Read the model definition and answer for the solid it produces. Units are mm, in the model's axes. Face numbers are marked on the shaded views. A direction names the side the tool comes from. Give positions to 0.01 mm unless a question says otherwise; leave off trailing zeros. Loops run counter-clockwise (first coordinate to the right, second up) from the corner with the lowest first, then second, coordinate; pieces in that order, holes last.
(1) Which of the six approach directions +Z, -Z, +X, -X, +Y, -Y give full straight-line access (tool end or side, diameter ignored) to the marked faces 1 and 2?
(2) Find section A-A, the plane z = 0. Write down the section's boundary in (x, y), then the cut area to 3 significant figures.
(3) Find section D-D, the plane x = 20. Write down the section's boundary in (y, z), then the cut area to 3 significant figures.
(4) Find section B-B, the plane x = 0. Write down the section's boundary in (y, z), then the cut area to 3 significant figures.
(5) Straight lines are drawn through the part: probe 1 along Y at (x, z) = (-24, -19); probe 2 along X at (y, z) = (8, 3.5); probe 3 along X at (y, z) = (8, -10). For each, find the intervals that lie inside material, in ascending order.
(6) Find section C-C, the plane y = 7.5. Write down the section's boundary in (x, z), then the cut area to 3 significant figures.
(7) This flat-tipped pin is pushed along its axis until it touches: P1, Ø2, axis at x = -23.5, z = -9.5, coming from the +Y side. Where does it stop, or does it pass through?
```python
from build123d import *

# Parameters (mm, degrees)
F0_W     = 65.434128046
F0_H     = 41.7352281511
F1_DEPTH = 25.4
F2_R     = 15.9425701821
F3_DEPTH = 7.366
F4_DEPTH = 0.254
F5_DEPTH = 3.302


with BuildPart() as f1:
    # F0 (on Front) → F1 (new body)
    with BuildSketch(Plane.XZ):
        Rectangle(F0_W, F0_H)
    extrude(amount=F1_DEPTH)

    # F2 (on face) → F3 (join)
    with BuildSketch(Plane(origin=(0, 0, 0), x_dir=(-1, 0, 0), z_dir=(0, 1, 0))):
        Circle(F2_R)
    extrude(amount=F3_DEPTH)

    # F4 (add): a face of the model
    f4_faces = [f1.faces().sort_by_distance(p)[0] for p in [
        (31.9409548566, 0, 0),
    ]]
    extrude(f4_faces, amount=F4_DEPTH)

    # F5 (add): a face of the model
    f5_faces = [f1.faces().sort_by_distance(p)[0] for p in [
        (0, 7.366, 0),
    ]]
    extrude(f5_faces, amount=F5_DEPTH)


solid = f1.part
```
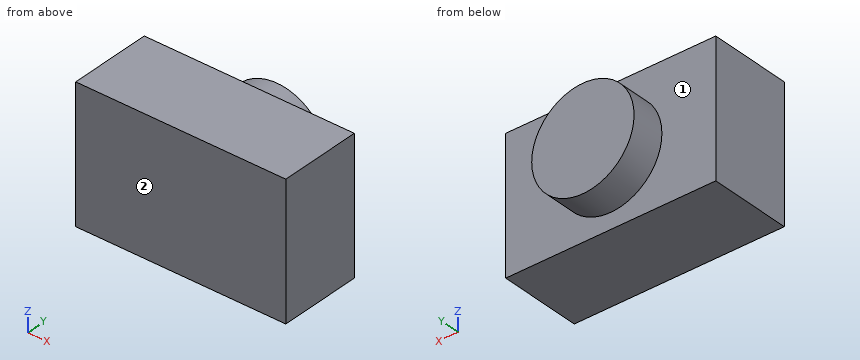
Entries:
1. face 1: +Y
1. face 2: +Z, -Z, +X, -X, -Y
2. outline: (-32.72, -25.4) - (32.72, -25.4) - (32.72, 0.25) - (15.94, 0.25) - (15.94, 10.67) - (-15.94, 10.67) - (-15.94, 0.25) - (-32.72, 0.25) - close
2. area: 2,010 mm2
3. outline: (-25.4, -20.87) - (0.25, -20.87) - (0.25, 20.87) - (-25.4, 20.87) - close
3. area: 1,070 mm2
4. outline: (-25.4, -20.87) - (0.25, -20.87) - (0.25, -15.94) - (10.67, -15.94) - (10.67, 15.94) - (0.25, 15.94) - (0.25, 20.87) - (-25.4, 20.87) - close
4. area: 1,400 mm2
5. probe 1: y = -25.4 to 0.25
5. probe 2: x = -15.55 to 15.55
5. probe 3: x = -12.42 to 12.42
6. outline: circle Ø31.89 at (0, 0)
6. area: 798 mm2
7. P1: stops at y = 0.25
